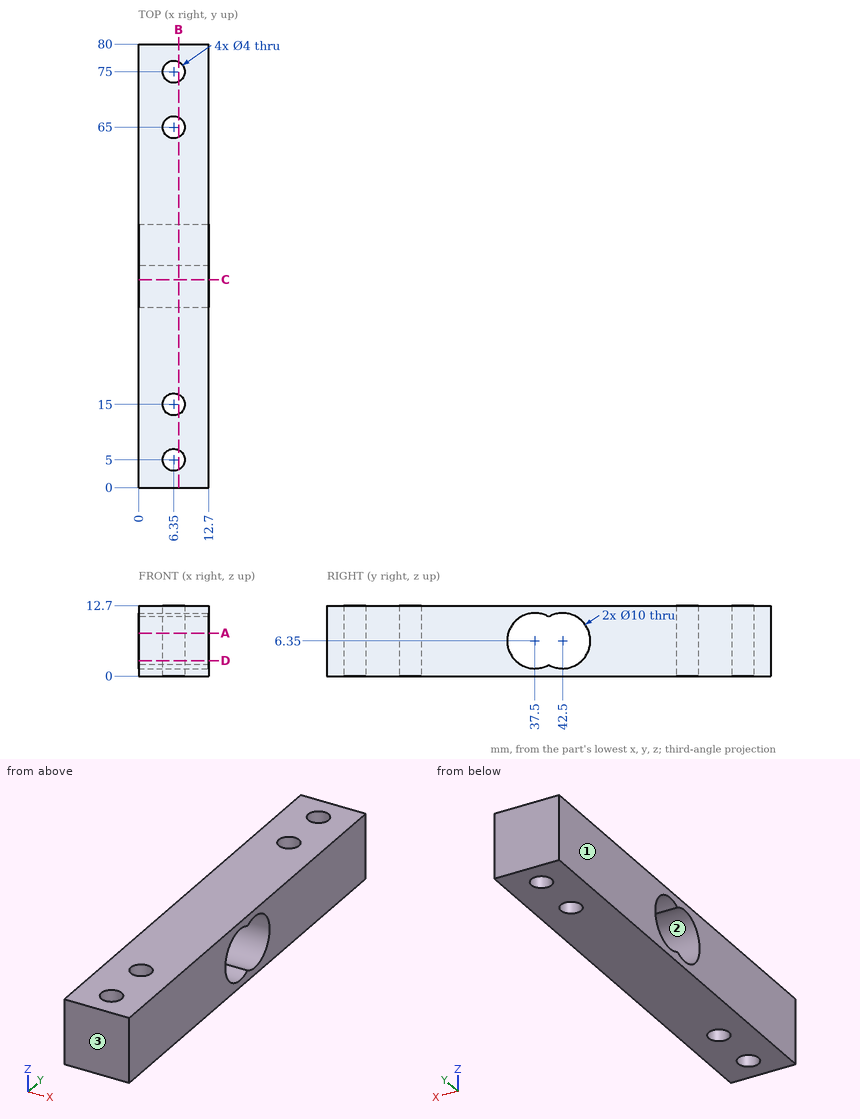
Verification items for this drawing (mm, ordinates from the low corner). Round coordinates to 2 decimals unless told otherwise and drop trailing zeros. Loops run counter-clockwise (first coordinate to the right, second up) from the corner with the lowest first, then second, coordinate; pieces in that order, holes last. Notation, with made-up numbers: M 68.25,83 L 117.25,83 A16 cw 117.25,96 Z; hole C 68,89 d7. An arc over 180 degrees is marked long. Answer as a JSON object with one key per item and string values.
1. Gauge pin test, flat end, axial feed: P1, Ø3, axis at x = 6.35, y = 5, coming from the +Z side. Record the tip position at first contact, or that the pin passes through.
Reply:
{"P1": "passes through"}
2. Section check D-D (z = 2.75). Record the boundary of the cut face in (x, y).
Reply:
{"outline": "M 0,0 L 12.7,0 L 12.7,34.03 L 0,34.03 Z; M 0,45.97 L 12.7,45.97 L 12.7,80 L 0,80 Z; hole C 6.35,5 d4; hole C 6.35,15 d4; hole C 6.35,65 d4; hole C 6.35,75 d4"}
3. Mould release check, pull along Y, two halves, no side actions. Record for the marked faces 1, 2 and 3: pulls with the +Y half, pulls with the -Y half, needs draft (parallel to the pull), parting line crosses it, or undercut.
Reply:
{"face 1": "needs draft", "face 2": "undercut", "face 3": "pulls with the -Y half"}
4. Scan lines: line 1 (Y direction, x = 6.35, z = 6.25); line 2 (Z direction, x = 5.75, y = 37.5); line 3 (Z direction, x = 12, y = 33). Record each from-to range of solid material in increasing order.
Reply:
{"line 1": "y = 0 to 3, 7 to 13, 17 to 32.5, 47.5 to 63, 67 to 73, 77 to 80", "line 2": "z = 0 to 1.35, 11.35 to 12.7", "line 3": "z = 0 to 4.17, 8.53 to 12.7"}
5. Section check C-C (y = 37.5). Record the boundary of the cut face in (x, z).
Reply:
{"outline": "M 0,0 L 12.7,0 L 12.7,1.35 L 0,1.35 Z; M 0,11.35 L 12.7,11.35 L 12.7,12.7 L 0,12.7 Z"}
6. Section check B-B (x = 7.25). Record the boundary of the cut face in (y, z).
Reply:
{"outline": "M 0,0 L 3.21,0 L 3.21,12.7 L 0,12.7 Z; M 6.79,0 L 13.21,0 L 13.21,12.7 L 6.79,12.7 Z; M 16.79,0 L 63.21,0 L 63.21,12.7 L 16.79,12.7 Z; M 66.79,0 L 73.21,0 L 73.21,12.7 L 66.79,12.7 Z; M 76.79,0 L 80,0 L 80,12.7 L 76.79,12.7 Z; hole M 40,2.02 A5 ccw long 40,10.68 A5 ccw long Z"}
7. Section check A-A (z = 7.75). Record the boundary of the cut face in (x, y), plus the area to 3 significant figures.
Reply:
{"outline": "M 0,0 L 12.7,0 L 12.7,32.7 L 0,32.7 Z; M 0,47.3 L 12.7,47.3 L 12.7,80 L 0,80 Z; hole C 6.35,5 d4; hole C 6.35,15 d4; hole C 6.35,65 d4; hole C 6.35,75 d4", "area": "780 mm²"}
